Here's how the part is built. I have some questions about the finished solid (model axes, mm). Face numbers are marked on the shaded views. A direction names the side the tool comes from. Coordinates: 2 decimals unless noted, no trailing zeros. Order: outer loops, then holes, each group sorted by start corner. A loop starts at its lowest first (then second) coordinate and runs counter-clockwise, first axis right, second up.
```python
from build123d import *

# Parameters (mm, degrees)
SKETCH1_R           = 1.651
BOSS_EXTRUDE1_DEPTH = 3.175
CUT_EXTRUDE2_DEPTH  = 6.35
SKETCH7_R           = 4.9784
SKETCH7_R_2         = 1.5875
CUT_EXTRUDE3_DEPTH  = 124.96234811
FILLET1_R           = 6.35
SKETCH8_W           = 50.8
SKETCH8_H           = 12.7
CUT_EXTRUDE4_DEPTH  = 50.8
CUT_EXTRUDE5_DEPTH  = 19.304
FILLET6_R           = 6.35
FILLET7_R           = 6.35
FILLET8_R           = 19.05
BOSS_EXTRUDE2_DEPTH = 3.175
FILLET9_R           = 24.13
SKETCH13_W          = 41.667851519
SKETCH13_H          = 9.459584315
SKETCH13_W_2        = 28.967851519
SKETCH13_H_2        = 8.468235606
BOSS_EXTRUDE3_DEPTH = 6.35
SKETCH16_R          = 4.09575
CUT_EXTRUDE8_DEPTH  = 137.155378763
BOSS_EXTRUDE4_DEPTH = 6.35
CUT_EXTRUDE9_DEPTH  = 119.214793194


with BuildPart() as part:
    # Sketch1 → Boss-Extrude1 (new body)
    with BuildSketch(Plane.XY):
        with BuildLine():
            Line((0, 0), (107.95, 0))
            Line((107.95, 0), (100.9362606, 26.175631792))
            Line((100.9362606, 26.175631792), (100.868755024, 26.427566033))
            ThreePointArc((100.868755024, 26.427566033), (110.348359368, 43.438223217), (95.367453293, 55.88))
            Line((95.367453293, 55.88), (0, 38.1))
            Line((0, 38.1), (0, 25.4))
            Line((0, 25.4), (-7.62, 25.4))
            Line((-7.62, 25.4), (-7.62, 12.7))
            Line((-7.62, 12.7), (0, 12.7))
            Line((0, 12.7), (0, 0))
        make_face()
        with Locations((25.817011896, 25.817011896)):
            Circle(SKETCH1_R, mode=Mode.SUBTRACT)
        with Locations((25.817011896, 12.282988104)):
            Circle(SKETCH1_R, mode=Mode.SUBTRACT)
        with Locations((12.282988104, 12.282988104)):
            Circle(SKETCH1_R, mode=Mode.SUBTRACT)
        with Locations((12.282988104, 25.817011896)):
            Circle(SKETCH1_R, mode=Mode.SUBTRACT)
    extrude(amount=BOSS_EXTRUDE1_DEPTH)

    # Sketch6 → Cut-Extrude2 (cut)
    with BuildSketch(Plane.XY.offset(3.175)):
        with BuildLine():
            Line((50.8, 0), (76.2, 0))
            ThreePointArc((76.2, 0), (63.5, 12.7), (50.8, 0))
        make_face()
    extrude(amount=-CUT_EXTRUDE2_DEPTH, mode=Mode.SUBTRACT)

    # Sketch7 → Cut-Extrude3 (cut, through all)
    with BuildSketch(Plane.XY.offset(3.175)):
        with Locations((19.05, 19.05)):
            Circle(SKETCH7_R)
        with Locations((80.766582748, 12.282988104)):
            Circle(SKETCH7_R_2)
        with Locations((94.299702748, 12.282988104)):
            Circle(SKETCH7_R_2)
        with Locations((80.766582748, 25.817011896)):
            Circle(SKETCH7_R_2)
        with Locations((94.299702748, 25.817011896)):
            Circle(SKETCH7_R_2)
    extrude(amount=-CUT_EXTRUDE3_DEPTH, mode=Mode.SUBTRACT)

    # Fillet1
    fillet1_edges = [part.edges().sort_by_distance(p)[0] for p in [
        (100.868755024, 26.427566033, 1.5875),
    ]]
    fillet(fillet1_edges, radius=FILLET1_R)

    # Sketch8 → Cut-Extrude4 (cut)
    with BuildSketch(Plane.XY.offset(3.175)):
        with Locations((25.4, 44.45)):
            Rectangle(SKETCH8_W, SKETCH8_H)
    extrude(amount=-CUT_EXTRUDE4_DEPTH, mode=Mode.SUBTRACT)

    # Sketch9 → Cut-Extrude5 (cut)
    with BuildSketch(Plane.XY.offset(3.175)):
        Polygon((50.8, 47.57098794), (50.8, 40.64), (57.15, 40.64), (57.15, 48.754861432), align=None)
    extrude(amount=-CUT_EXTRUDE5_DEPTH, mode=Mode.SUBTRACT)

    # Fillet6
    fillet6_edges = [part.edges().sort_by_distance(p)[0] for p in [
        (57.15, 40.64, 1.5875),
    ]]
    fillet(fillet6_edges, radius=FILLET6_R - 0.0001)  # a hair under: the kernel refuses the full size

    # Fillet7
    fillet7_edges = [part.edges().sort_by_distance(p)[0] for p in [
        (57.15, 48.754861432, 1.5875),
    ]]
    fillet(fillet7_edges, radius=FILLET7_R)

    # Fillet8
    fillet8_edges = [part.edges().sort_by_distance(p)[0] for p in [
        (50.8, 0, 1.5875),
    ]]
    fillet(fillet8_edges, radius=FILLET8_R)

    # Sketch12 → Boss-Extrude2 (add)
    with BuildSketch(Plane.XY.offset(3.175)):
        with BuildLine():
            Line((50.8, 40.64), (85.027112904, 40.64))
            Line((85.027112904, 40.64), (95.367453293, 55.88))
            add(Edge.make_bspline(
                [(50.8, 40.64), (70.777788932, 52.178803671), (78.594281742, 111.543427795), (95.367453293, 55.88)],
                knots=[0, 0, 0, 0, 1, 1, 1, 1], degree=3))
        make_face()
    extrude(amount=-BOSS_EXTRUDE2_DEPTH)

    # Fillet9
    fillet9_edges = [part.edges().sort_by_distance(p)[0] for p in [
        (95.367453293, 55.88, 1.5875),
    ]]
    fillet(fillet9_edges, radius=FILLET9_R)

    # Sketch13 → Boss-Extrude3 (add)
    with BuildSketch(Plane(origin=(0, 0, 0), x_dir=(-1, 0, 0), z_dir=(0, 0, -1))):
        with Locations((-29.966074241, 33.370207843)):
            Rectangle(SKETCH13_W, SKETCH13_H)
        with Locations((-23.616074241, 4.234117803)):
            Rectangle(SKETCH13_W_2, SKETCH13_H_2)
    extrude(amount=-BOSS_EXTRUDE3_DEPTH)

    # Sketch16 → Cut-Extrude8 (cut, through all)
    with BuildSketch(Plane.XY.offset(3.175)):
        with Locations((89.473702748, 46.137011896)):
            Circle(SKETCH16_R)
    extrude(amount=-CUT_EXTRUDE8_DEPTH, mode=Mode.SUBTRACT)

    # Sketch18 → Boss-Extrude4 (add)
    with BuildSketch(Plane.XY.offset(3.175)):
        Polygon((0, 0), (7.62, 0), (7.62, 38.1), (0, 38.1), (0, 25.4), (-7.62, 25.4), (-7.62, 12.7), (0, 12.7), align=None)
    extrude(amount=-BOSS_EXTRUDE4_DEPTH)

    # Sketch19 → Cut-Extrude9 (cut, through all)
    with BuildSketch(Plane(origin=(0, 38.1, 0), x_dir=(1, 0, 0), z_dir=(0, 1, 0))):
        Polygon((9.132148481, -3.175), (12.307148481, -6.35), (9.132148481, -6.35), align=None)
    extrude(amount=-CUT_EXTRUDE9_DEPTH, mode=Mode.SUBTRACT)


solid = part.part
```
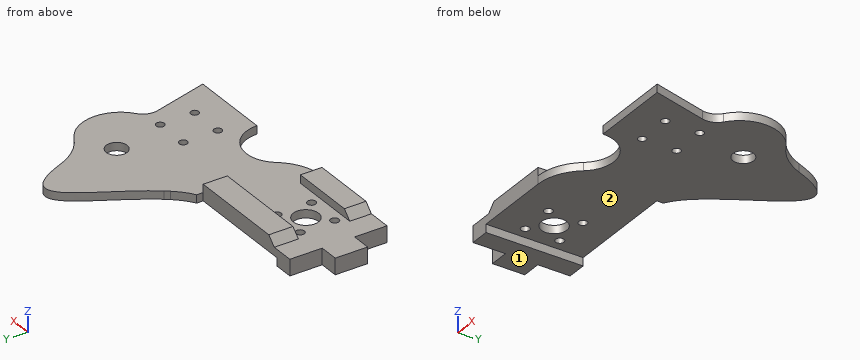
Q1. If we section it at C-C on x = 47.5: Write out the boundary of the cut face in (y, z) (3 decimals), then the cut area to 3 significant figures.
Q2. If we section it at D-D on y = 33.5: Write out the boundary of the cut face in (x, z) (3 decimals).
Q3. Will these pins go through, and if not, where does the flat tip stop? pin 1 (5 mm diameter, centred on x = 80.77, y = 12.28, fed in from -Z); pin 2 (1 mm diameter, centred on x = 17.5, z = 5.5, fed in from +Y); pin 3 (4 mm diameter, centred on y = 57.5, z = -1, fed in from -X).
Q4. If we section it at B-B on y = 20.5: Write out the boundary of the cut face in (x, z) (3 decimals).
Q5. For the marked faces 1 and 2, which set-ups out of +Z, -Z, +X, -X, +Y, -Y let a thin tool reach every point of the face, with its end or its side?
Q6. If we section it at A-A on x = 19.05: Write out the boundary of the cut face in (y, z) (3 decimals), then the cut area to 3 significant figures.
Q7. I need wall thicknesses on L1, parallel to X at y = 13, z = 2.25; L2, parallel to Y at x = 36, z = 5.5; L3, parallel to Z at x = 8, y = 23.5 (3 decimals). Which ranges of each line are inside material? Lowest first, please.
Reply:
1. outline: (2.481, 0) - (38.1, 0) - (38.1, 6.35) - (28.64, 6.35) - (28.64, 3.175) - (2.481, 3.175) - close
1. area: 143 mm2
2. outline: (0, -3.175) - (7.62, -3.175) - (7.62, 0) - (108.831, 0) - (108.831, 3.175) - (50.8, 3.175) - (50.8, 6.35) - (12.307, 6.35) - (9.132, 3.175) - (0, 3.175) - close
3. pin 1: stops at z = 0
3. pin 2: stops at y = 38.1
3. pin 3: stops at x = 63.86
4. outline: (-7.62, -3.175) - (7.62, -3.175) - (7.62, 0) - (14.287, 0) - (14.287, 3.175) - (-7.62, 3.175) - close; (23.813, 0) - (102.457, 0) - (102.457, 3.175) - (23.813, 3.175) - close
5. face 1: -Z, +X, -X, +Y, -Y
5. face 2: -Z, +X, +Y, -Y
6. outline: (0, 0) - (14.072, 0) - (14.072, 3.175) - (8.468, 3.175) - (8.468, 6.35) - (0, 6.35) - close; (24.028, 0) - (38.1, 0) - (38.1, 6.35) - (28.64, 6.35) - (28.64, 3.175) - (24.028, 3.175) - close
6. area: 146 mm2
7. L1: x = -7.62 to 10.8, 13.77 to 24.33, 27.3 to 79.35, 82.18 to 92.88, 95.72 to 104.47
7. L2: y = 0 to 8.47, 28.64 to 38.1
7. L3: z = 0 to 3.175
